Verification items for the finished model (mm, model axes). Face numbers are marked on the shaded views. Give positions to 0.01 mm unless a question says otherwise; leave off trailing zeros. Loops run counter-clockwise (first coordinate to the right, second up) from the corner with the lowest first, then second, coordinate; pieces in that order, holes last. Notation, with made-up numbers: (57.5, 89.25) - (106.5, 89.25) arc R28 cw to (106.5, 113.25) - close; hole circle Ø10 at (67, 63). An arc over 180 degrees is marked (long way). Use one line per item in the form item = value.
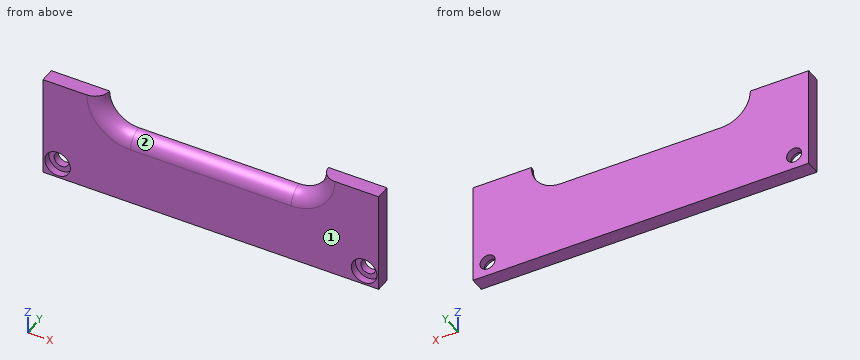
Autodesk Inventor part; units mm, degrees
ref_plane "YZ Plane" through (0, 0, 0) normal (1, 0, 0) x (0, 1, 0)
ref_plane "XZ Plane" through (0, 0, 0) normal (0, 1, 0) x (-1, 0, 0)
ref_plane "XY Plane" through (0, 0, 0) normal (0, 0, 1) x (1, 0, 0)
sketch "Sketch1" plane through (0, 0, 0) normal (0, 1, 0) x (-1, 0, 0)
  line L0 (0, 0) -> (73.025, 0)
  line L1 (73.025, 0) -> (73.025, -22.225)
  line L2 (73.025, -22.225) -> (0, -22.225)
  line L3 (0, -22.225) -> (0, 0)
  line L4 (73.025, 0) -> (53.975, 0)
  line L5 (0, 0) -> (19.05, 0)
  line L6 (53.975, 0) -> (19.05, 0) construction
  line L7 (53.975, 6.35) -> (19.05, 6.35)
  line L8 (19.05, -6.35) -> (53.975, -6.35)
  arc A0 (53.975, -6.35) -> (53.975, 6.35) centre (53.975, 0) ccw
  arc A1 (19.05, 6.35) -> (19.05, -6.35) centre (19.05, 0) ccw
  line L9 (73.025, -22.225) -> (69.85, -22.225)
  line L10 (69.85, -22.225) -> (69.85, -19.05)
  line L11 (69.85, -19.05) -> (73.025, -19.05)
  line L12 (73.025, -19.05) -> (73.025, -22.225)
  line L13 (0, -22.225) -> (3.175, -22.225)
  line L14 (3.175, -22.225) -> (3.175, -19.05)
  line L15 (3.175, -19.05) -> (0, -19.05)
  line L16 (0, -19.05) -> (0, -22.225)
  point P0 (36.5125, 0)
  point P1 (60.325, 0)
  point P2 (12.7, 0)
  dimension "d0" = 73.025
  dimension "d1" = 22.225
  dimension "d2" = 19.05
  dimension "d3" = 19.05
  dimension "d4" = 12.7
  dimension "d7" = 3.175
  dimension "d8" = 3.175
  dimension "d9" = 3.175
  dimension "d10" = 3.175
extrude "Extrusion1" add sketch "Sketch1" along normal blind 3.175 contours A1 L8 A0 L0 L1 L11 L10 L2 L14 L15 L3 | L15 L14 L2 L3 | L1 L2 L10 L11
hole "Hole1" at (-69.85, 0, -19.05) at (-3.175, 0, -19.05) direction (0, 1, 0) diameter 3.2766 end through all counterbore diameter 5.5626 counterbore depth 1.5875
fillet "Fillet2" radius 3.175 3 edges at (-14.5599, 0, -4.4901) (-58.4651, 0, -4.4901) (-36.5125, 0, -6.35)
properties part number "Compute Module Top Cover for RoadBot Rail-r1"
1. Depth check by flat-ended pin: pin 1 Ø10 at (x, z) = (-37, -3.5) entering from -Y; pin 2 Ø1 at (x, y) = (-33, 2) entering from +Z. Enter the tip coordinate at first touch or a pass-through.
Result set:
pin_1 = 0.17
pin_2 = -6.42
2. Draft check along X on the marked faces 1 and 2. Enter one of: released by +X, released by -X, zero draft, split by the parting line, or undercut.
Result set:
face_1 = zero draft
face_2 = undercut
3. Section check A-A, the plane z = -19.05. State how many separate pieces and enclosed holes the cut face has, then the cut area to 3 significant figures.
Result set:
separate_pieces = 3
enclosed_holes = 0
area = 204 mm²
4. Scan lines: probe 1 along X at (y, z) = (2.8, -19.05) (3 decimals); probe 2 along X at (y, z) = (0.8, -19.05) (3 decimals); probe 3 along Z at (x, y) = (-69.85, 1.25) (3 decimals). Record each from-to range of solid material in increasing order.
Result set:
probe_1 = -73.025 to -71.488, -68.212 to -4.813, -1.537 to 0
probe_2 = -73.025 to -72.631, -67.069 to -5.956, -0.394 to 0
probe_3 = -22.225 to -21.831, -16.269 to 0
5. Section check C-C, the plane y = 1. Record the cut outline in (x, z) (3 decimals).
Result set:
outline = (-73.025, -22.225) - (0, -22.225) - (0, 0) - (-11.838, 0) arc R7.212 cw to (-19.05, -7.212) - (-53.975, -7.212) arc R7.212 cw to (-61.187, 0) - (-73.025, 0) - close; hole circle Ø5.563 at (-69.85, -19.05); hole circle Ø5.563 at (-3.175, -19.05)
